```python
from build123d import *

# Parameters (mm, degrees)
F1_DEPTH         = 10
F3_D             = 2.05
F4_D             = 3
F4_DEPTH         = 5
F4_TIP           = 0.9012909285
F5_R             = 6
F7_DEPTH         = 24.751
F8_R             = 1
F10_D            = 2.9464
F10_DEPTH        = 5
F10_TIP          = 0.885187864
F12_D            = 2.2606
F12_DEPTH        = 5
F12_TIP          = 0.6791527577
F15_D            = 2.7051
F15_DEPTH        = 7
F15_TIP          = 0.8126940303
F15_ON_F14_D     = 2.7051
F15_ON_F14_DEPTH = 7
F15_ON_F14_TIP   = 0.8126940303


with BuildPart() as f1:
    # F0 (on Top) → F1 (new body)
    with BuildSketch(Plane.XY):
        with BuildLine():
            Line((0, 35), (0, 0))
            Line((0, 0), (35, 0))
            Line((35, 0), (35, 10.25))
            Line((35, 10.25), (60, 10.25))
            Line((60, 10.25), (60, 15.25))
            Line((60, 15.25), (40, 15.25))
            ThreePointArc((40, 15.25), (37.75, 17.5), (40, 19.75))
            Line((40, 19.75), (60, 19.75))
            Line((60, 19.75), (60, 24.75))
            Line((60, 24.75), (35, 24.75))
            Line((35, 24.75), (35, 35))
            Line((35, 35), (0, 35))
        make_face()
    extrude(amount=F1_DEPTH)

    # F3 (through all)
    with Locations(Plane.XY.offset(10)):
        with Locations((3, 32), (32, 32), (32, 3), (3, 3)):
            Hole(F3_D / 2)

    # F4
    with Locations(Plane.XY.offset(10)):
        with Locations((10.5, 31), (24.5, 4)):
            Hole(F4_D / 2, depth=F4_DEPTH)
            with Locations((0, 0, -(F4_DEPTH + F4_TIP / 2))):  # 118° drill point
                Cone(0, F4_D / 2, F4_TIP, mode=Mode.SUBTRACT)

    # F5
    f5_edges = [f1.edges().sort_by_distance(p)[0] for p in [
        (35, 10.25, 5),
        (35, 24.75, 5),
    ]]
    fillet(f5_edges, radius=F5_R)

    # F6 (on face) → F7 (cut, through all)
    with BuildSketch(Plane.XZ.offset(-10.25)):
        with BuildLine():
            Line((43, 7), (60, 7))
            Line((60, 7), (60, 10))
            Line((60, 10), (41, 10))
            Line((41, 10), (41, 9))
            ThreePointArc((41, 9), (41.5857864376, 7.5857864376), (43, 7))
        make_face()
    extrude(amount=-F7_DEPTH, mode=Mode.SUBTRACT)

    # F8
    f8_edges = [f1.edges().sort_by_distance(p)[0] for p in [
        (60, 12.75, 7),
        (60, 22.25, 7),
        (60, 22.25, 0),
        (60, 12.75, 0),
    ]]
    fillet(f8_edges, radius=F8_R)

    # F10
    with Locations(Plane(origin=(0, 24.75, 0), x_dir=(-1, 0, 0), z_dir=(0, 1, 0))):
        with Locations((-57, 3.75)):
            Hole(F10_D / 2, depth=F10_DEPTH)
            with Locations((0, 0, -(F10_DEPTH + F10_TIP / 2))):  # 118° drill point
                Cone(0, F10_D / 2, F10_TIP, mode=Mode.SUBTRACT)

    # F12
    with Locations(Plane.XZ.offset(-10.25)):
        with Locations((57, 3.75)):
            Hole(F12_D / 2, depth=F12_DEPTH)
            with Locations((0, 0, -(F12_DEPTH + F12_TIP / 2))):  # 118° drill point
                Cone(0, F12_D / 2, F12_TIP, mode=Mode.SUBTRACT)

    # F15
    with Locations(Plane(origin=(0, 35, 0), x_dir=(-1, 0, 0), z_dir=(0, 1, 0))):
        with Locations((-17.5, 5)):
            Hole(F15_D / 2, depth=F15_DEPTH)
            with Locations((0, 0, -(F15_DEPTH + F15_TIP / 2))):  # 118° drill point
                Cone(0, F15_D / 2, F15_TIP, mode=Mode.SUBTRACT)

    # F15 on F14
    with Locations(Plane.XZ):
        with Locations((17.5, 5)):
            Hole(F15_ON_F14_D / 2, depth=F15_ON_F14_DEPTH)
            with Locations((0, 0, -(F15_ON_F14_DEPTH + F15_ON_F14_TIP / 2))):  # 118° drill point
                Cone(0, F15_ON_F14_D / 2, F15_ON_F14_TIP, mode=Mode.SUBTRACT)


solid = f1.part
```
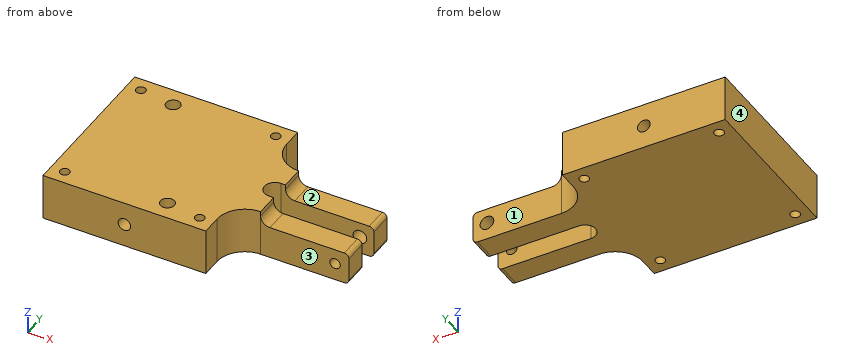
Verification items for the finished model (mm, model axes). Face numbers are marked on the shaded views. A direction names the side the tool comes from. Coordinates: 2 decimals unless noted, no trailing zeros. Write each loop counter-clockwise with the first axis right and the second up, starting at its lowest first coordinate (ties: lowest second). Pieces come first, ordered by that corner, then holes. Notation, with made-up numbers: M 37,59 L 70,59 A30 cw 70,97 Z; hole C 29,84.5 d9. An arc over 180 degrees is marked long. Answer as a JSON object with one key per item and string values. Group by question number.
(1) Cross-section at B-B, the plane x = 47.5. Record the cut outline in (y, z).
(2) Tool access check on the marked faces 1, 2, 3 and 4. Record the directions out of +Z, -Z, +X, -X, +Y, -Y that give a thin tool (end or side, any length) a straight path to the whole face; none if there is none.
(3) Material ranges on line 1 (Y direction, x = 32, z = 7.5) (3 decimals); line 2 (Y direction, x = 53, z = 6.5); line 3 (Y direction, x = 24.5, z = 8.7), recorded low to high.
(4) Cross-section at C-C, the plane y = 17.5. Record the cut outline in (x, z).
(5) Cross-section at A-A, the plane x = 32. Record the cut outline in (y, z) (3 decimals).
(6) Gauge pin test, flat ends, axial feed: pin 1 (1.8 mm diameter, centred on x = 57, z = 3.75, fed in from +Y); pin 2 (4 mm diameter, centred on y = 7, z = 8.5, fed in from +X); pin 3 (5.5 mm diameter, centred on x = 49.5, y = 21.5, fed in from +Z); pin 4 (2 mm diameter, centred on y = 32.5, z = 3.5, fed in from +X). Record the tip position at first contact, or that the pin passes through.
Reply:
{
 "1": {"outline": "M 10.25,0 L 15.25,0 L 15.25,7 L 10.25,7 Z; M 19.75,0 L 24.75,0 L 24.75,7 L 19.75,7 Z"},
 "2": {"face 1": "+Z, -Z, +X, +Y", "face 2": "+Z, +X, +Y, -Y", "face 3": "+Z, -Z, +X, -Y", "face 4": "+Z, -Z, -X, +Y, -Y"},
 "3": {"line 1": "0 to 1.975, 4.025 to 30.975, 33.025 to 35", "line 2": "10.25 to 15.25, 19.75 to 24.75", "line 3": "0 to 2.5, 5.5 to 35"},
 "4": {"outline": "M 0,0 L 37.75,0 L 37.75,10 L 0,10 Z"},
 "5": {"outline": "M 0,0 L 1.975,0 L 1.975,10 L 0,10 Z; M 4.025,0 L 30.975,0 L 30.975,10 L 4.025,10 Z; M 33.025,0 L 35,0 L 35,10 L 33.025,10 Z"},
 "6": {"pin 1": "through", "pin 2": "x = 37.33", "pin 3": "z = 7", "pin 4": "x = 35"}
}
